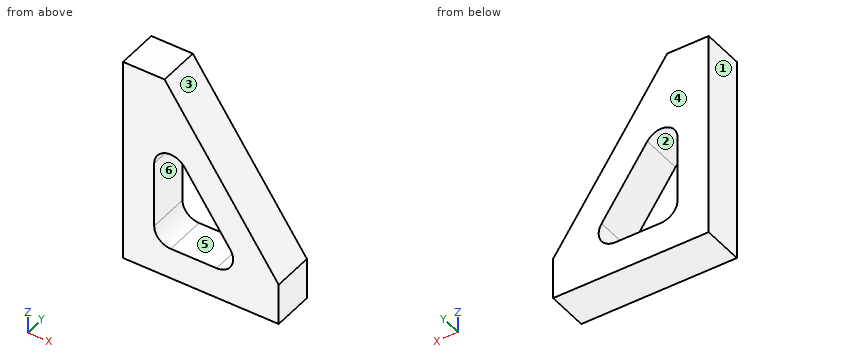
```python
from build123d import *

# Parameters (mm, degrees)
F4_DEPTH = 25.4


with BuildPart() as f4:
    # F3 (on Front) → F4 (new body)
    with BuildSketch(Plane.XZ):
        Polygon((0, 61.356521979), (-25.4, 61.356521979), (-25.4, -65.643478021), (69.85, -65.643478021), (69.85, -40.243478021), align=None)
        with BuildLine():
            ThreePointArc((-6.35, 4.2551029085), (0.7964159254, 13.9578814293), (12.1822659499, 10.011035749))
            Line((12.1822659499, 10.011035749), (40.1556653389, -30.6775451805))
            ThreePointArc((40.1556653389, -30.6775451805), (40.7752256123, -41.1634527747), (31.783399389, -46.593478021))
            Line((31.783399389, -46.593478021), (3.81, -46.593478021))
            ThreePointArc((3.81, -46.593478021), (-3.3742048969, -43.6176829179), (-6.35, -36.433478021))
            Line((-6.35, -36.433478021), (-6.35, 4.2551029085))
        make_face(mode=Mode.SUBTRACT)
    extrude(amount=F4_DEPTH)


solid = f4.part
```
CAD build for the part. Positions are in the model's coordinates, mm. Face numbers are marked on the shaded views. A direction names the side the tool comes from. Round coordinates to 2 decimals unless told otherwise and drop trailing zeros. Order: outer loops, then holes, each group sorted by start corner. A loop starts at its lowest first (then second) coordinate and runs counter-clockwise, first axis right, second up.
Q1. Slice it at C-C (x = 17). Write the cut outline in (y, z), and give its area (3 significant figures).
Q2. Two-plate mould, pull along Z, no slides. Class the marked faces 3, 4, 5 and 6: pulls with the +Z half, pulls with the -Z half, needs draft (parallel to the pull), parting line crosses it, or undercut.
Q3. Which spindle directions (+Z, -Z, +X, -X, +Y, -Y) get a long thin tool onto all of the face, cutting with end or side? Do the marked faces 1 and 2. Say none if no direction does.
Q4. Drop flat-ended pins along their axis: pin 1 (10 mm diameter, centred on x = 18.5, z = 48.5, fed in from +Y); pin 2 (2 mm diameter, centred on y = -21.5, z = -30, fed in from +X); pin 3 (4 mm diameter, centred on y = -20.5, z = -24.5, fed in from +X); pin 4 (8 mm diameter, centred on x = 35.5, y = -22, fed in from +Z). Give the stop position or say it passes through.
Q5. Wall check: L1, parallel to X at y = -2.5, z = -38; L2, parallel to X at y = -2.25, z = -13; L3, parallel to Z at x = 36, y = -22.75. Give the ranges that are in metal, low to high.
Q6. Slice it at D-D (z = 50.5). Write the cut outline in (x, y), and give its area (3 significant figures).
Q7. Slice it at A-A (y = -16.5). Write the cut outline in (x, z), and give its area (3 significant figures).
Q8. Slice it at B-B (z = -26). Write the cut outline in (x, y), and give its area (3 significant figures).
Results below:
1. outline: (-25.4, -65.64) - (0, -65.64) - (0, -46.59) - (-25.4, -46.59) - close; (-25.4, 3) - (0, 3) - (0, 36.63) - (-25.4, 36.63) - close
1. area: 1,340 mm2
2. face 3: pulls with the +Z half
2. face 4: needs draft
2. face 5: undercut
2. face 6: undercut
3. face 1: +Z, -Z, -X, +Y, -Y
3. face 2: +Y, -Y
4. pin 1: passes through
4. pin 2: stops at x = 63.5
4. pin 3: stops at x = 60.4
4. pin 4: stops at z = 15.54
5. L1: x = -25.4 to -6.23, 41.82 to 68.31
5. L2: x = -25.4 to -6.35, 28 to 51.12
5. L3: z = -65.64 to -45.68, -24.63 to 8.99
6. outline: (-25.4, -25.4) - (7.46, -25.4) - (7.46, 0) - (-25.4, 0) - close
6. area: 835 mm2
7. outline: (-25.4, -65.64) - (69.85, -65.64) - (69.85, -40.24) - (0, 61.36) - (-25.4, 61.36) - close; hole (-6.35, -36.43) arc R10.16 ccw to (3.81, -46.59) - (31.78, -46.59) arc R10.16 ccw to (40.16, -30.68) - (12.18, 10.01) arc R10.16 ccw to (-6.35, 4.26) - close
7. area: 6,460 mm2
8. outline: (-25.4, -25.4) - (-6.35, -25.4) - (-6.35, 0) - (-25.4, 0) - close; (36.94, -25.4) - (60.06, -25.4) - (60.06, 0) - (36.94, 0) - close
8. area: 1,070 mm2
